```python
from build123d import *

# Parameters (mm, degrees)
FILLET_1_R = 0.25


with BuildPart() as part:
    # Эскиз1 → Повернуть1 (revolve)
    with BuildSketch(Plane(origin=(0, 0, 0), x_dir=(0, 0, -1), z_dir=(1, 0, 0)), mode=Mode.PRIVATE) as revolve_1_sk:
        Polygon((23, 0), (35, 0), (35, 5), (34, 5), (33.5, 4.5), (23.5, 4.5), (23, 5), (9.5, 5), (9.5, 4.5), (8.75, 4.5), (8.75, 5), (0, 5), (0, 3.75), (23, 3.75), align=None)
    revolve(revolve_1_sk.sketch.rotate(Axis((0, 0, -23), (0, 0, -1)), 90), axis=Axis((0, 0, -23), (0, 0, -1)))

    # Скругление1
    fillet_1_edges = [part.edges().sort_by_distance(p)[0] for p in [
        (-3.75, 0, 0),
        (-5, 0, 0),
    ]]
    fillet(fillet_1_edges, radius=FILLET_1_R)


solid = part.part
```
CAD build for the part. Positions are in the model's coordinates, mm. A direction names the side the tool comes from. Coordinates: 2 decimals unless noted, no trailing zeros. Loops run counter-clockwise (first coordinate to the right, second up) from the corner with the lowest first, then second, coordinate; pieces in that order, holes last. Notation, with made-up numbers: (84.5, 25.25) - (118.5, 25.25) arc R8 ccw to (118.5, 38.25) - close; hole circle Ø3 at (84, -30). An arc over 180 degrees is marked (long way). Use CSV: the item, a comma, the result in double quotes. Start each with the question number.
Q1. 3-axis set-ups, long thin cutter, end or side, ignore diameter. For faces 4 (the flat face through (0, 0, -23)), 5 (the cylindrical face through (-3.32, -3.04, -9.12)), 6 (the cylindrical face through (-5, 0, -16)): which of +Z, -Z, +X, -X, +Y, -Y reach the whole face in a straight line?
Q2. Drop flat-ended pins along their axis: P1, Ø5, axis at y = -2.5, z = -13.5, coming from the +X side; P2, Ø4, axis at y = -3, z = -17.5, coming from the +X side; P3, Ø1.5, axis at x = 2.5, z = -26, coming from the -Y side; P4, Ø1.5, axis at y = -1, z = -30.5, coming from the -X side. Give the stop position or say it passes through.
Q3. Cut at A-A, the plane y = 0. List the corners of the cut face in (x, z).
Q4. Probe probe 1 along Z at (x, y) = (-2.75, -3.75); probe 2 along Y at (x, z) = (0, -6.25); probe 3 along Z at (x, y) = (0, 0.5). List the from-to ranges inside material, lowest first. Write a range as from..to.
Q5. Cut at C-C, the plane z = -12. List the corners of the cut face in (x, y).
Q6. Two-plate mould, pull along Z, no slides. Class faces 1 (the flat face through (-4, 2, 0)), 2 (the cylindrical face through (2.02, -3.16, -11.78)), 3 (the cylindrical face through (-3.32, -3.04, -28.43)): +Z half, -Z half, draft (parallel to the pull), parting line (faces both ways), or undercut.
Q7. Cut at D-D, the plane z = -31. List the corners of the cut face in (x, y), then the cut area to 3 significant figures.
Here are the results:
1,face 4,"+Z"
1,face 5,"none"
1,face 6,"+Z, -Z"
2,P1,"x = 5"
2,P2,"x = 4.9"
2,P3,"y = -4.15"
2,P4,"x = -4.49"
3,outline,"(-5, -35) - (5, -35) - (5, -34) - (4.5, -33.5) - (4.5, -23.5) - (5, -23) - (5, -9.5) - (4.5, -9.5) - (4.5, -8.75) - (5, -8.75) - (5, -0.25) arc R0.25 ccw to (4.75, 0) - (4, 0) arc R0.25 ccw to (3.75, -0.25) - (3.75, -23) - (-3.75, -23) - (-3.75, -0.25) arc R0.25 ccw to (-4, 0) - (-4.75, 0) arc R0.25 ccw to (-5, -0.25) - (-5, -8.75) - (-4.5, -8.75) - (-4.5, -9.5) - (-5, -9.5) - (-5, -23) - (-4.5, -23.5) - (-4.5, -33.5) - (-5, -34) - close"
4,probe 1,"-35..-33.65, -23.35..-9.5, -8.75..0"
4,probe 2,"-5..-3.75, 3.75..5"
4,probe 3,"-35..-23"
5,outline,"circle Ø10 at (0, 0); hole circle Ø7.5 at (0, 0)"
6,face 1,"+Z half"
6,face 2,"draft"
6,face 3,"undercut"
7,outline,"circle Ø9 at (0, 0)"
7,area,"63.6 mm2"
